The listing builds one solid part. Answer for the finished solid, in the listing's coordinates (mm). Face numbers are marked on the shaded views. Give positions to 0.01 mm unless a question says otherwise; leave off trailing zeros. One line per item, written item: value. Start each with the question number.
from build123d import *

# Parameters (mm, degrees)
BOSS_EXTRUDE1_DEPTH = 1000
CUT_EXTRUDE3_DEPTH  = 100
SKETCH3_6_R         = 1.5
SKETCH3_6_R_2       = 2.5
SKETCH3_6_R_3       = 1.501016752
CUT_EXTRUDE4_DEPTH  = 100


with BuildPart() as part:
    # Sketch1 → Boss-Extrude1 (new body)
    with BuildSketch(Plane.XY):
        Polygon((11.571428571, 55), (11.571428571, 7), (3, 7), (3, 55), (0, 55), (0, 7), (0, 0), (165, 0), (165, 7), (165, 10), (165, 55), (162, 55), (162, 7), (153.428571429, 7), (153.428571429, 55), (150.428571429, 55), (150.428571429, 7), (141.857142857, 7), (141.857142857, 55), (138.857142857, 55), (138.857142857, 7), (130.285714286, 7), (130.285714286, 55), (127.285714286, 55), (127.285714286, 7), (118.714285714, 7), (118.714285714, 55), (115.714285714, 55), (115.714285714, 7), (107.142857143, 7), (107.142857143, 55), (104.142857143, 55), (104.142857143, 7), (95.571428571, 7), (95.571428571, 55), (92.571428571, 55), (92.571428571, 7), (84, 7), (84, 55), (81, 55), (81, 7), (72.428571429, 7), (72.428571429, 55), (69.428571429, 55), (69.428571429, 7), (60.857142857, 7), (60.857142857, 55), (57.857142857, 55), (57.857142857, 7), (49.285714286, 7), (49.285714286, 55), (46.285714286, 55), (46.285714286, 7), (37.714285714, 7), (37.714285714, 55), (34.714285714, 55), (34.714285714, 7), (26.142857143, 7), (26.142857143, 55), (23.142857143, 55), (23.142857143, 7), (14.571428571, 7), (14.571428571, 55), align=None)
    extrude(amount=BOSS_EXTRUDE1_DEPTH)

    # Sketch3 → Cut-Extrude3 (cut)
    with BuildSketch(Plane.XZ):
        with BuildLine():
            Line((135.172029065, 203.361980458), (132.300867592, 192.646659963))
            ThreePointArc((132.300867592, 192.646659963), (126.177143235, 189.111126057), (122.641609329, 195.234850414))
            Line((122.641609329, 195.234850414), (125.512770802, 205.950170909))
            ThreePointArc((125.512770802, 205.950170909), (98, 217.952595893), (73.849209656, 235.778141844))
            Line((73.849209656, 235.778141844), (66.005050634, 227.933982822))
            ThreePointArc((66.005050634, 227.933982822), (58.933982822, 227.933982822), (58.933982822, 235.005050634))
            Line((58.933982822, 235.005050634), (66.778141844, 242.849209656))
            ThreePointArc((66.778141844, 242.849209656), (48.952595893, 267), (36.950170909, 294.512770802))
            Line((36.950170909, 294.512770802), (26.234850414, 291.641609329))
            ThreePointArc((26.234850414, 291.641609329), (20.111126057, 295.177143235), (23.646659963, 301.300867592))
            Line((23.646659963, 301.300867592), (34.361980458, 304.172029065))
            ThreePointArc((34.361980458, 304.172029065), (31.843147719, 318.991579341), (31, 334))
            Line((31, 334), (165, 334))
            Line((165, 334), (165, 1000))
            Line((165, 1000), (0, 1000))
            Line((0, 1000), (0, 0))
            Line((0, 0), (165, 0))
            Line((165, 0), (165, 200))
            ThreePointArc((165, 200), (149.991579341, 200.843147719), (135.172029065, 203.361980458))
        make_face()
    extrude(amount=-CUT_EXTRUDE3_DEPTH, mode=Mode.SUBTRACT)

    # Sketch3<6> → Cut-Extrude4 (cut)
    with BuildSketch(Plane.XZ):
        with Locations((117, 236)):
            Circle(SKETCH3_6_R)
        with Locations((106.834, 241.544)):
            Circle(SKETCH3_6_R)
        with Locations((127.47123846, 193.940755188)):
            Circle(SKETCH3_6_R_2)
        with Locations((62.469516728, 231.469516728)):
            Circle(SKETCH3_6_R_2)
        with Locations((24.940755188, 296.47123846)):
            Circle(SKETCH3_6_R_2)
        with Locations((159, 206)):
            Circle(SKETCH3_6_R)
        with Locations((159.945, 224.958)):
            Circle(SKETCH3_6_R)
        with Locations((138.59, 236)):
            Circle(SKETCH3_6_R)
        with Locations((107, 220)):
            Circle(SKETCH3_6_R)
        with Locations((92.864, 261.61)):
            Circle(SKETCH3_6_R)
        with Locations((74.576, 273.548)):
            Circle(SKETCH3_6_R)
        with Locations((68.48, 283.2)):
            Circle(SKETCH3_6_R)
        with Locations((51, 276)):
            Circle(SKETCH3_6_R)
        with Locations((152.097, 291.028)):
            Circle(SKETCH3_6_R)
        with Locations((133.3, 304.5)):
            Circle(SKETCH3_6_R)
        with Locations((66.702, 306.822)):
            Circle(SKETCH3_6_R)
        with Locations((56.542, 323.078)):
            Circle(SKETCH3_6_R)
        with Locations((38, 327)):
            Circle(SKETCH3_6_R)
        with Locations((124, 325)):
            Circle(SKETCH3_6_R)
        with Locations((158, 321)):
            Circle(SKETCH3_6_R_3)
        with Locations((151.6, 326.9)):
            Circle(SKETCH3_6_R)
    extrude(amount=-CUT_EXTRUDE4_DEPTH, mode=Mode.SUBTRACT)


solid = part.part
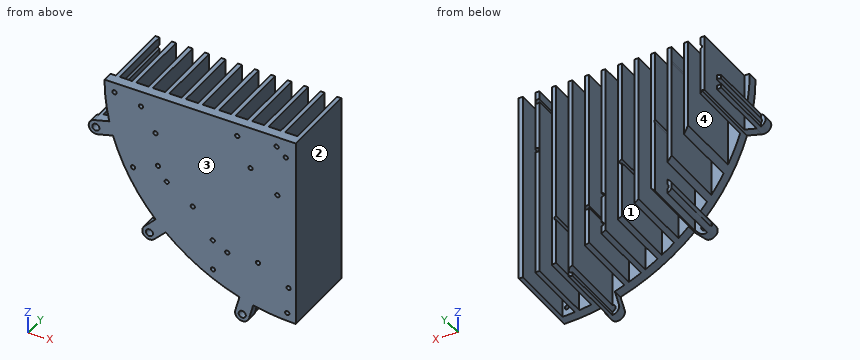
Item 1: Each of these flat-tipped pins is pushed along its axis until it touches: pin 1 Ø12 at (y, z) = (23.5, 304.5) entering from -X; pin 2 Ø4 at (x, z) = (124, 325) entering from +Y; pin 3 Ø24 at (y, z) = (25, 264) entering from -X. Where does it stop, or does it pass through?
Item 2: The mould has two halves that part along X. Classify the marked faces 1, 2, 3 and 4: +X half, -X half, draft (parallel to the pull), parting line (faces both ways), or undercut.
Item 3: Find section A-A on y = 19. Give the number of separate pieces and of enclosed holes in the cut face, plus the area to 3 significant figures.
Item 4: Straight lines are drawn through the part: line 1 along Y through (x, z) = (91.5, 232.5); line 2 along X through (y, z) = (9, 199.5); line 3 along Z through (x, y) = (128.5, 7). For each, find the intervals that lie inside material, in ascending order.
Values:
1. pin 1: x = 23.14
1. pin 2: y = 7
1. pin 3: x = 46.29
2. face 1: undercut
2. face 2: +X half
2. face 3: draft
2. face 4: undercut
3. separate pieces: 15
3. enclosed holes: 0
3. area: 3,880 mm^2
4. line 1: 0 to 7
4. line 2: 127.29 to 130.29
4. line 3: 189.05 to 191.66, 196.22 to 334
